from build123d import *

# Parameters (mm, degrees)
ESQUISSE1_W                  = 270
ESQUISSE1_H                  = 75
BOSS_EXTRU_1_DEPTH           = 5
ESQUISSE2_R                  = 2
ENL_V_MAT_EXTRU_1_DEPTH      = 141.200748928
ENL_V_MAT_EXTRU_2_DEPTH      = 141.200748928
ENL_V_MAT_EXTRU_2_DEPTH_BACK = 141.200748928
ESQUISSE4_W                  = 270
ESQUISSE4_H                  = 5
ENL_V_MAT_EXTRU_3_DEPTH      = 30


with BuildPart() as part:
    # Esquisse1 → Boss.-Extru.1 (new body)
    with BuildSketch(Plane.XY):
        Rectangle(ESQUISSE1_W, ESQUISSE1_H)
    extrude(amount=BOSS_EXTRU_1_DEPTH)

    # Esquisse2 → Enlèv. mat.-Extru.1 (cut, through all)
    with BuildSketch(Plane.XY.offset(5)):
        with Locations((123, 0.5)):
            Circle(ESQUISSE2_R)
        with Locations((123, -14.5)):
            Circle(ESQUISSE2_R)
        with Locations((-123, 4.5)):
            Circle(ESQUISSE2_R)
        with Locations((-123, -9.5)):
            Circle(ESQUISSE2_R)
    extrude(amount=-ENL_V_MAT_EXTRU_1_DEPTH, mode=Mode.SUBTRACT)

    # Esquisse3 → Enlèv. mat.-Extru.2 (cut, two sides: drawn at the far end of the back side and taken through both)
    with BuildSketch(Plane.XY.offset(5).offset(-ENL_V_MAT_EXTRU_2_DEPTH_BACK)):
        with BuildLine():
            Line((-98, -37.5), (-62, -37.5))
            ThreePointArc((-62, -37.5), (-60.585786438, -36.914213562), (-60, -35.5))
            Line((-60, -35.5), (-60, -19.5))
            ThreePointArc((-60, -19.5), (-60.585786438, -18.085786438), (-62, -17.5))
            Line((-62, -17.5), (-98, -17.5))
            ThreePointArc((-98, -17.5), (-99.414213562, -18.085786438), (-100, -19.5))
            Line((-100, -19.5), (-100, -35.5))
            ThreePointArc((-100, -35.5), (-99.414213562, -36.914213562), (-98, -37.5))
        make_face()
        with BuildLine():
            ThreePointArc((-54.387545621, -31.3), (-58.25, -32.6), (-54.387545621, -33.9))
            ThreePointArc((-54.387545621, -33.9), (-53.95, -32.6), (-54.387545621, -31.3))
        make_face()
        with BuildLine():
            ThreePointArc((-54.387545621, -21.1), (-58.25, -22.4), (-54.387545621, -23.7))
            ThreePointArc((-54.387545621, -23.7), (-53.95, -22.4), (-54.387545621, -21.1))
        make_face()
        with BuildLine():
            ThreePointArc((-105.612454379, -33.9), (-101.75, -32.6), (-105.612454379, -31.3))
            ThreePointArc((-105.612454379, -31.3), (-106.05, -32.6), (-105.612454379, -33.9))
        make_face()
        with BuildLine():
            ThreePointArc((-105.612454379, -23.7), (-101.75, -22.4), (-105.612454379, -21.1))
            ThreePointArc((-105.612454379, -21.1), (-106.05, -22.4), (-105.612454379, -23.7))
        make_face()
    extrude(amount=ENL_V_MAT_EXTRU_2_DEPTH + ENL_V_MAT_EXTRU_2_DEPTH_BACK, mode=Mode.SUBTRACT)

    # Esquisse4 → Enlèv. mat.-Extru.3 (cut)
    with BuildSketch(Plane(origin=(0, 37.5, 0), x_dir=(1, 0, 0), z_dir=(0, 1, 0))):
        with Locations((0, -2.5)):
            Rectangle(ESQUISSE4_W, ESQUISSE4_H)
    extrude(amount=-ENL_V_MAT_EXTRU_3_DEPTH, mode=Mode.SUBTRACT)


solid = part.part
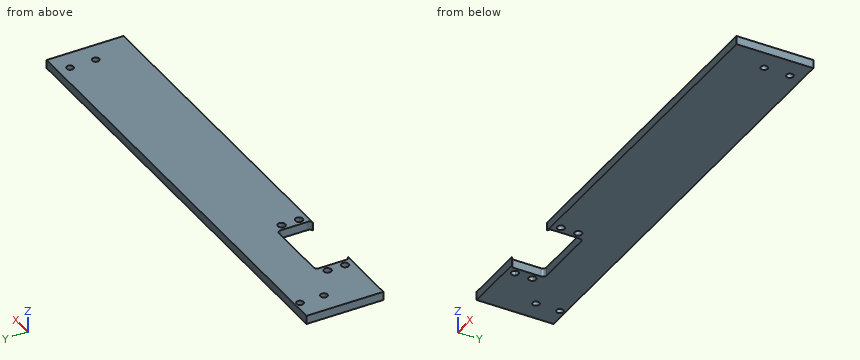
For this review, take the finished solid that the model builds, in its own axes (mm). Give positions to 0.01 mm unless a question says otherwise; leave off trailing zeros. Loops run counter-clockwise (first coordinate to the right, second up) from the corner with the lowest first, then second, coordinate; pieces in that order, holes last.
Item 1: Insertion check: pin 1 (1.5 mm diameter, centred on x = -75, z = 1.5, fed in from -Y). The pin has a flat end and moves straight along its axis. Give the tip position at first contact, or say it passes through.
Item 2: Take a section at B-B, the plane x = -84.5. State the section outline as (y, z) points, and give its area (3 significant figures).
Item 3: Take a section at A-A, the plane z = 1.35. Give the number of separate pieces and of enclosed holes in the cut face, and give its area (3 significant figures).
Item 4: For line 1 along Y through (x, z) = (-123, 3.55); line 2 along Y through (x, z) = (-103.9, 1.9); line 3 along X through (y, z) = (-33, 3.8), list the stretches that pass through material, from the lowest coordinate up.
Calculated:
1. pin 1: stops at y = -17.5
2. outline: (-17.5, 0) - (7.5, 0) - (7.5, 5) - (-17.5, 5) - close
2. area: 125 mm2
3. separate pieces: 1
3. enclosed holes: 8
3. area: 11,200 mm2
4. line 1: y = -37.5 to -11.5, -7.5 to 2.5, 6.5 to 7.5
4. line 2: y = -37.5 to -34.75, -30.45 to -24.55, -20.25 to 7.5
4. line 3: x = -135 to -106.01, -101.79 to -100, -60 to -58.21, -53.99 to 135
